Answer from the drawing. Dimensions are ordinates in mm from the lowest x, y and z of the part. A direction names the side the tool comes from. Give positions to 0.01 mm unless a question says otherwise; leave off trailing zeros. Order: outer loops, then holes, each group sorted by start corner. A loop starts at its lowest first (then second) coordinate and runs counter-clockwise, first axis right, second up.
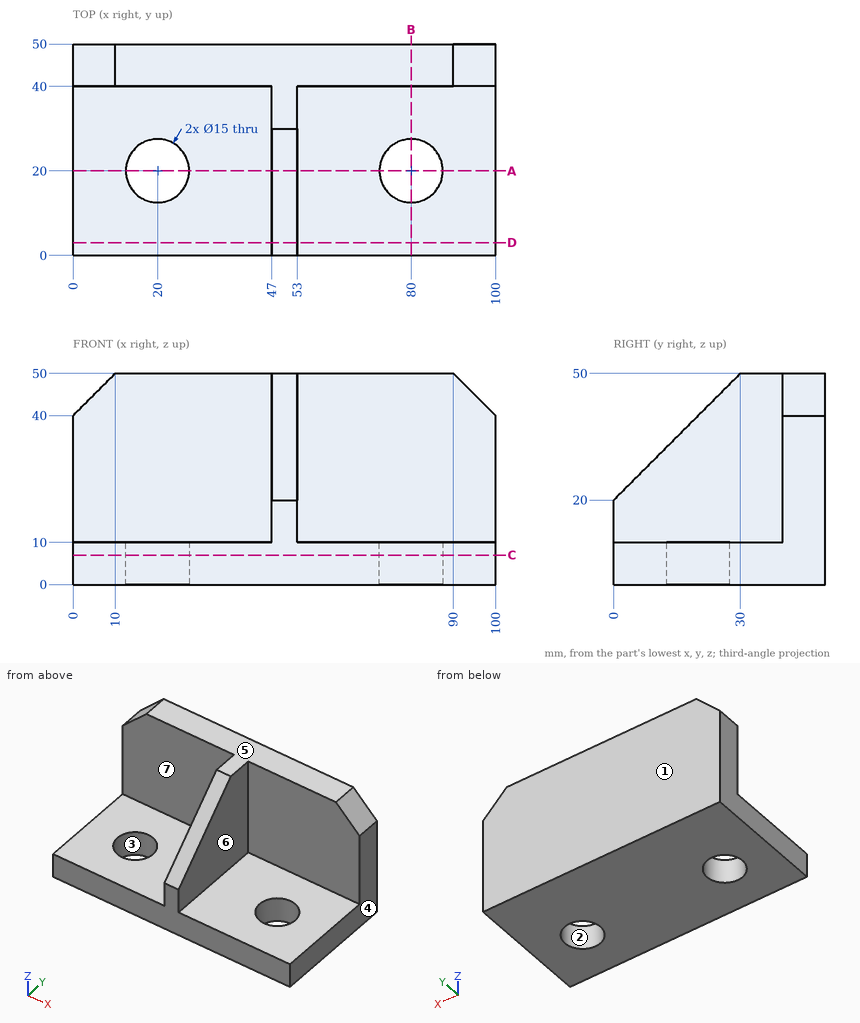
1. The part is cut by section A-A (y = 20). Write down the section's boundary in (x, z), then the cut area to 3 significant figures.
Findings below:
outline: (0, 0) - (12.5, 0) - (12.5, 10) - (0, 10) - close; (27.5, 0) - (72.5, 0) - (72.5, 10) - (53, 10) - (53, 40) - (47, 40) - (47, 10) - (27.5, 10) - close; (87.5, 0) - (100, 0) - (100, 10) - (87.5, 10) - close
area: 880 mm2
2. The part is cut by section C-C (z = 7). Write down the section's boundary in (x, y), then the cut area to 3 significant figures.
Findings below:
outline: (0, 0) - (100, 0) - (100, 50) - (0, 50) - close; hole circle Ø15 at (20, 20); hole circle Ø15 at (80, 20)
area: 4,650 mm2
3. The mould has two halves that part along Y. Classify the marked faces 1, 2, 3 and 4: pulls with the +Y half, pulls with the -Y half, needs draft (parallel to the pull), parting line crosses it, or undercut.
Findings below:
face 1: pulls with the +Y half
face 2: undercut
face 3: undercut
face 4: needs draft
4. Given P1, Ø2, axis at y = 23.5, z = 12.5, coming from the -X side; P2, Ø10, axis at x = 44, y = 35.5, coming from the -Z side; P3, Ø1.5, axis at y = 8.5, z = 23.5, coming from the +X side; P4, Ø20, axis at x = 67.5, z = 29, coming from the -Y side, each flat-ended and moving along its own axis, determine where each tip first touches the part or whether it passes through.
Findings below:
P1: stops at x = 47
P2: stops at z = 0
P3: stops at x = 53
P4: stops at y = 40
5. The part is cut by section D-D (y = 3). Write down the section's boundary in (x, z), then the cut area to 3 significant figures.
Findings below:
outline: (0, 0) - (100, 0) - (100, 10) - (53, 10) - (53, 23) - (47, 23) - (47, 10) - (0, 10) - close
area: 1,080 mm2
6. Straight lines are drawn through the part: probe 1 along Y at (x, z) = (20, 5); probe 2 along Y at (x, z) = (88, 15); probe 3 along X at (y, z) = (37.5, 29). For each, find the intervals that lie inside material, in ascending order.
Findings below:
probe 1: y = 0 to 12.5, 27.5 to 50
probe 2: y = 40 to 50
probe 3: x = 47 to 53
7. Which of the six approach directions +Z, -Z, +X, -X, +Y, -Y give full straight-line access (tool end or side, diameter ignored) to the marked faces 5, 6 and 7?
Findings below:
face 5: +Z, +X, -X, +Y, -Y
face 6: +Z, +X, -Y
face 7: +Z, -X, -Y
8. The part is cut by section B-B (x = 80). Write down the section's boundary in (y, z).
Findings below:
outline: (0, 0) - (12.5, 0) - (12.5, 10) - (0, 10) - close; (27.5, 0) - (50, 0) - (50, 50) - (40, 50) - (40, 10) - (27.5, 10) - close
